Read the model definition and answer for the solid it produces. Units are mm, in the model's axes. A direction names the side the tool comes from. Coordinates: 2 decimals unless noted, no trailing zeros. Write each loop counter-clockwise with the first axis right and the second up, starting at its lowest first coordinate (ties: lowest second). Pieces come first, ordered by that corner, then holes. Notation, with made-up numbers: (58, 88.25) -> (73, 88.25) arc R19 ccw to (73, 122.25) -> close; hole circle Ø3 at (-31.5, 29.5). An arc over 180 degrees is marked (long way). One line per item, written item: value. Start each with the question number.
from build123d import *

# Parameters (mm, degrees)
SKETCH2_R           = 10
BOSS_EXTRUDE1_DEPTH = 15
SKETCH3_R           = 7.5
BOSS_EXTRUDE2_DEPTH = 10
SKETCH8_R           = 7.5
BOSS_EXTRUDE3_DEPTH = 30
SKETCH4_W           = 35
SKETCH4_H           = 315
SKETCH9_W           = 70
SKETCH9_H           = 80
CUT_EXTRUDE1_DEPTH  = 15


with BuildPart() as part:
    # Sketch1 → Base-Revolve (revolve)
    with BuildSketch(Plane.XY, mode=Mode.PRIVATE) as base_revolve_sk:
        Polygon((22.5, -330), (40, -330), (40, -10), (45, -10), (45, 40), (50, 40), (50, 70), (0, 70), (0, 55), (35, 55), (35, -325), (22.5, -325), align=None)
    revolve(base_revolve_sk.sketch.rotate(Axis((0, 100, 0), (0, -1, 0)), 90), axis=Axis((0, 100, 0), (0, -1, 0)))

    # Sketch2 → Boss-Extrude1 (add, symmetric)
    with BuildSketch(Plane.XY):
        with BuildLine():
            Line((19.138857956, 105.805524623), (30, 70))
            Line((30, 70), (-30, 70))
            Line((-30, 70), (-19.138857956, 105.805524623))
            ThreePointArc((-19.138857956, 105.805524623), (0, 120), (19.138857956, 105.805524623))
        make_face()
        with Locations((0, 100)):
            Circle(SKETCH2_R, mode=Mode.SUBTRACT)
    extrude(amount=BOSS_EXTRUDE1_DEPTH, both=True)

    # Sketch3 → Boss-Extrude2 (add, symmetric)
    with BuildSketch(Plane.XY):
        with BuildLine():
            Line((62.373967528, -280.189048708), (30, -275))
            Line((30, -275), (30, -315))
            Line((30, -315), (62.373967528, -309.810951292))
            ThreePointArc((62.373967528, -309.810951292), (75, -295), (62.373967528, -280.189048708))
        make_face()
        with Locations((60, -295)):
            Circle(SKETCH3_R, mode=Mode.SUBTRACT)
    boss_extrude2 = extrude(amount=BOSS_EXTRUDE2_DEPTH, both=True)

    # Mirror1: Boss-Extrude2 across plane
    add(boss_extrude2.mirror(Plane(origin=(0, 0, 0), x_dir=(0, 0, 1), z_dir=(1, 0, 0))))

    # Sketch8 → Boss-Extrude3 (add, symmetric)
    with BuildSketch(Plane.XY):
        with BuildLine():
            Line((82.041582998, -85.08350067), (20, -80))
            Line((20, -80), (20, -140))
            Line((20, -140), (82.041582998, -134.91649933))
            ThreePointArc((82.041582998, -134.91649933), (105, -110), (82.041582998, -85.08350067))
        make_face()
        with Locations(Location((80, -110, 0), (0, 0, 180))):
            Circle(SKETCH8_R, mode=Mode.SUBTRACT)
    extrude(amount=BOSS_EXTRUDE3_DEPTH, both=True)

    # Sketch4 → Cut-Revolve1 (revolve, cut)
    with BuildSketch(Plane.XY):
        with Locations((17.5, -167.5)):
            Rectangle(SKETCH4_W, SKETCH4_H)
    revolve(axis=Axis((0, 0, 0), (0, -1, 0)), mode=Mode.SUBTRACT)

    # Sketch9 → Cut-Extrude1 (cut, symmetric)
    with BuildSketch(Plane.XY):
        with Locations((90, -110)):
            Rectangle(SKETCH9_W, SKETCH9_H)
    extrude(amount=CUT_EXTRUDE1_DEPTH, both=True, mode=Mode.SUBTRACT)


solid = part.part
1. A cutting plane is placed at C-C on y = 100. Give the vertices of the cut face in (x, z).
2. A tool of negligible diameter and unlimited length cuts with its end or side. For faces 1 (the face through (0.4, 89.8, -15)), 2 (the face through (-1, 70, 22)), 3 (the face through (56, -110, 30)), 4 (the face through (-53, -299, -10)), from which of +Z, -Z, +X, -X, +Y, -Y can it reach the whole face along a straight path? Write none if from no direction.
3. A cutting plane is placed at B-B on x = 0. Give the vertices of the cut face in (y, z).
4. A cutting plane is placed at D-D on y = -295. Give the vertices of the cut face in (x, z).
5. Find the intervals of material crossed by probe 1 along X at (y, z) = (-77, 0); probe 2 along Z at (x, y) = (2.5, 18); probe 3 along Y at (x, z) = (0, 7.5), in increasing order. Write a range as from..to.
6. For a pull along Z with two mould halves and no side action, classify faces 5 (the face through (-53, -299, 10)), 6 (the face through (34.168, -137.66, -7.587)), 7 (the face through (74, -116, 15)), 8 (the face through (26.5, -10, 30.2)) as +Z half, -Z half, draft (parallel to the pull), parting line (faces both ways), or undercut.
7. A cutting plane is placed at A-A on y = -110. Give the vertices of the cut face in (x, z), then the cut area to 3 significant figures.
8. Given pin 1 (1.5 mm diameter, centred on y = -178, z = -10.5, fed in from +X); pin 2 (2 mm diameter, centred on x = -40, y = 10.5, fed in from +Z); pin 3 (25 mm diameter, centred on x = 12, y = 92.5, fed in from -Z), each flat-ended and moving along its own axis, determine where each tip first touches the part or whether it passes through.
Derived:
1. outline: (-20.9, -15) -> (-10, -15) -> (-10, 15) -> (-20.9, 15) -> close; (10, -15) -> (20.9, -15) -> (20.9, 15) -> (10, 15) -> close
2. face 1: -Z, +X, -X, +Y
2. face 2: +Y
2. face 3: +Z, +X, -Y
2. face 4: -Z, -X, -Y
3. outline: (-330, -40) -> (-10, -40) -> (-10, -45) -> (40, -45) -> (40, -50) -> (70, -50) -> (70, -15) -> (90, -15) -> (90, 15) -> (70, 15) -> (70, 50) -> (40, 50) -> (40, 45) -> (-10, 45) -> (-10, 40) -> (-330, 40) -> (-330, 22.5) -> (-325, 22.5) -> (-325, 35) -> (55, 35) -> (55, -35) -> (-325, -35) -> (-325, -22.5) -> (-330, -22.5) -> close; (110, -15) -> (120, -15) -> (120, 15) -> (110, 15) -> close
4. outline: (-75, -10) -> (-67.5, -10) -> (-67.5, 10) -> (-75, 10) -> close; (-52.5, -10) -> (-38.73, -10) arc R40 ccw to (38.73, -10) -> (52.5, -10) -> (52.5, 10) -> (38.73, 10) arc R40 ccw to (-38.73, 10) -> (-52.5, 10) -> close; (67.5, -10) -> (75, -10) -> (75, 10) -> (67.5, 10) -> close; hole circle Ø70 at (0, 0)
5. probe 1: x = -40..-35, 35..40
5. probe 2: z = -44.93..-34.91, 34.91..44.93
5. probe 3: y = 55..90, 110..120
6. face 5: +Z half
6. face 6: undercut
6. face 7: undercut
6. face 8: draft
7. outline: (26.46, -30) -> (72.5, -30) -> (72.5, -15) -> (55, -15) -> (55, 15) -> (72.5, 15) -> (72.5, 30) -> (26.46, 30) arc R40 ccw (long way) to start; (87.5, -30) -> (105, -30) -> (105, -15) -> (87.5, -15) -> close; (87.5, 15) -> (105, 15) -> (105, 30) -> (87.5, 30) -> close; hole circle Ø70 at (0, 0)
7. area: 3,380 mm2
8. pin 1: stops at x = 38.79
8. pin 2: stops at z = 22.45
8. pin 3: stops at z = -15
